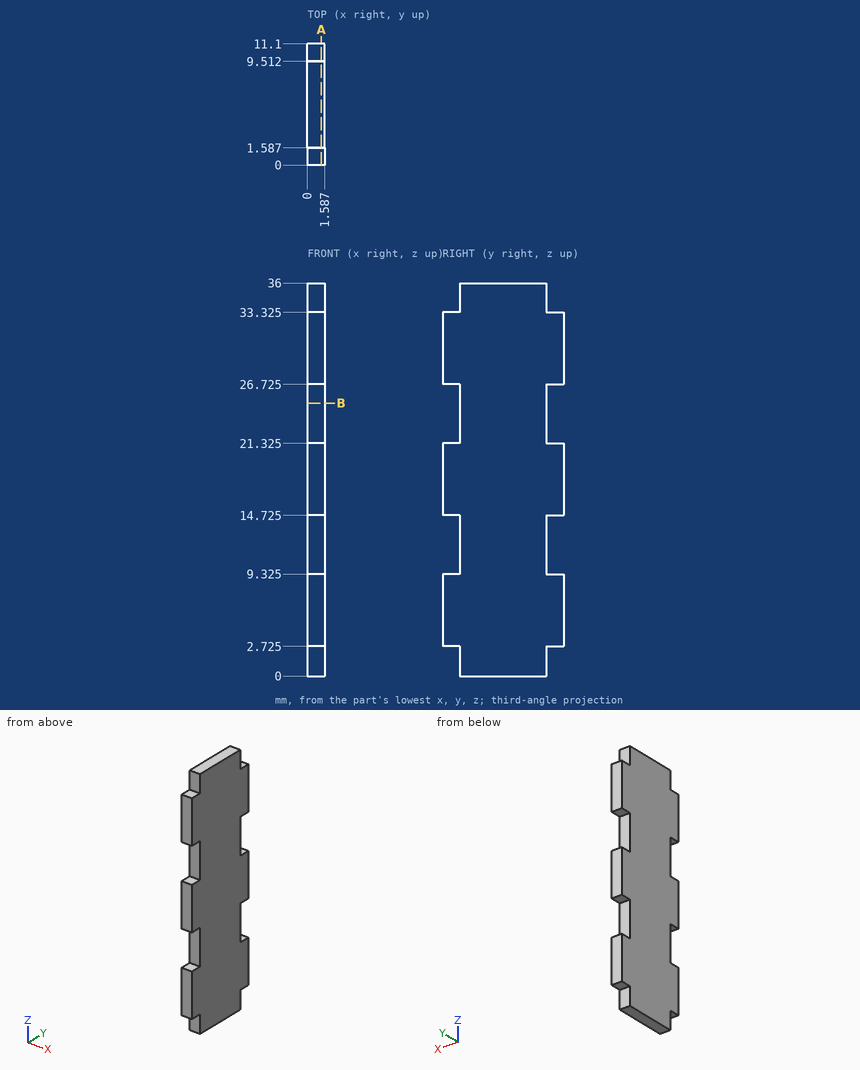
Can you work these out from the drawing? Everything is in mm from the part's minimum corner. Coordinates: 2 decimals unless noted, no trailing zeros. Loops run counter-clockwise (first coordinate to the right, second up) from the corner with the lowest first, then second, coordinate; pieces in that order, holes last. Notation, with made-up numbers: (67.25, 42) - (122.25, 42) arc R20 cw to (122.25, 55) - close; hole circle Ø2 at (-24, 75). An arc over 180 degrees is marked (long way). Answer as CSV lines item,"result".
Q1. If we section it at A-A, the plane x = 1.3: Write out the boundary of the cut face in (y, z) (1 decimal).
Response:
outline,"(0, 2.7) - (1.6, 2.7) - (1.6, 0) - (9.5, 0) - (9.5, 2.7) - (11.1, 2.7) - (11.1, 9.3) - (9.5, 9.3) - (9.5, 14.7) - (11.1, 14.7) - (11.1, 21.3) - (9.5, 21.3) - (9.5, 26.7) - (11.1, 26.7) - (11.1, 33.3) - (9.5, 33.3) - (9.5, 36) - (1.6, 36) - (1.6, 33.3) - (0, 33.3) - (0, 26.7) - (1.6, 26.7) - (1.6, 21.3) - (0, 21.3) - (0, 14.7) - (1.6, 14.7) - (1.6, 9.3) - (0, 9.3) - close"
Q2. For pin 1 (0.8 mm diameter, centred on x = 0.5, y = 0.5, fed in from +Z) (1 decimal); pin 2 (4 mm diameter, centred on y = 2, z = 7.5, fed in from -X); pin 3 (0.8 mm diameter, centred on x = 1, y = 1, fed in from -Z) (1 decimal); pin 4 (0.8 mm diameter, centred on x = 1, z = 1.5, fed in from -Y), each with a flat end and sliding along its axis, tell me the tip position at first contact or that it passes through.
Response:
pin 1,"z = 33.3"
pin 2,"x = 0"
pin 3,"z = 2.7"
pin 4,"y = 1.59"
Q3. If I drill on L1, parallel to Z at x = 1.2, y = 0.5 (1 decimal); L2, parallel to Y at x = 0.5, z = 2, over which ranges is the centre line in solid material (lowest first)? Write a range as [from, to].
Response:
L1,"[2.7, 9.3], [14.7, 21.3], [26.7, 33.3]"
L2,"[1.59, 9.51]"
Q4. If we section it at B-B, the plane z = 25: Write out the boundary of the cut face in (x, y), and give its area (3 significant figures).
Response:
outline,"(0, 1.59) - (1.59, 1.59) - (1.59, 9.51) - (0, 9.51) - close"
area,"12.6 mm2"
